Source: CAD feature listing. Evaluate the final solid. Frame: model axes, mm. A direction names the side the tool comes from. Give positions to 0.01 mm unless a question says otherwise; leave off trailing zeros. Order: outer loops, then holes, each group sorted by start corner. A loop starts at its lowest first (then second) coordinate and runs counter-clockwise, first axis right, second up. Notation, with made-up numbers: (35, 0.5) -> (75, 0.5) arc R30 ccw to (75, 30.5) -> close; hole circle Ø5 at (-37.75, -33). An arc over 180 degrees is marked (long way). Answer in a Markdown table with one row per item.
```python
from build123d import *

# Parameters (mm, degrees)
F0_W     = 57.15
F0_H     = 44.45
F1_DEPTH = 25.4
F2_W     = 44.45
F2_H     = 31.75
F3_DEPTH = 25.401
F5_DEPTH = 12.701
F7_DEPTH = 25.4


with BuildPart() as f1:
    # F0 (on Front) → F1 (new body)
    with BuildSketch(Plane.XZ):
        with Locations((-6.2023242936, 14.8889736688)):
            Rectangle(F0_W, F0_H)
    extrude(amount=F1_DEPTH)

    # F2 (on face) → F3 (cut, through all)
    with BuildSketch(Plane.XZ.offset(25.4)):
        with Locations((0.1476757064, 21.2389736688)):
            Rectangle(F2_W, F2_H)
    extrude(amount=-F3_DEPTH, mode=Mode.SUBTRACT)

    # F4 (on face) → F5 (cut, through all)
    with BuildSketch(Plane.XY.offset(5.3639736688)):
        with BuildLine():
            ThreePointArc((16.0226757064, -12.7), (14.1628037685, -8.209871941), (9.6726757108, -6.35))
            Line((9.6726757064, -6.35), (9.6726757064, -12.7))
            Line((9.6726757064, -12.7), (9.6726757064, -19.05))
            ThreePointArc((9.6726757179, -19.05), (14.162803771, -17.1901280565), (16.0226757064, -12.7))
        make_face()
        with BuildLine():
            ThreePointArc((9.6726757108, -6.35), (5.1825476475, -8.2098719379), (3.3226757064, -12.7))
            ThreePointArc((3.3226757064, -12.7), (5.18254765, -17.1901280646), (9.6726757179, -19.05))
            Line((9.6726757064, -19.05), (9.6726757064, -12.7))
            Line((9.6726757064, -12.7), (9.6726757064, -6.35))
        make_face()
        with BuildLine():
            ThreePointArc((-9.3773242936, -6.35), (-13.8674523541, -8.2098719395), (-15.7273242936, -12.7))
            ThreePointArc((-15.7273242936, -12.7), (-13.8674523541, -17.1901280605), (-9.3773242936, -19.05))
            ThreePointArc((-9.3773242936, -19.05), (-4.887196233, -17.1901280605), (-3.0273242936, -12.7))
            ThreePointArc((-3.0273242936, -12.7), (-4.887196233, -8.2098719395), (-9.3773242936, -6.35))
        make_face()
        with BuildLine():
            Line((16.0226757064, 0), (16.0226757064, -1.7014773719))
            ThreePointArc((16.0226757064, -1.7014773719), (18.6529318275, -3.7197438789), (20.6711983345, -6.35))
            Line((20.6711983345, -6.35), (22.3726757064, -6.35))
            Line((22.3726757064, -6.35), (22.3726757064, 0))
            Line((22.3726757064, 0), (16.0226757064, 0))
        make_face()
        with BuildLine():
            Line((16.0226757064, 0), (9.6726757064, 0))
            ThreePointArc((9.6726757064, 0), (12.9596775792, -0.4327420061), (16.0226757064, -1.7014773719))
            Line((16.0226757064, -1.7014773719), (16.0226757064, 0))
        make_face()
        with BuildLine():
            Line((22.3726757064, -6.35), (20.6711983345, -6.35))
            ThreePointArc((20.6711983345, -6.35), (21.9399337003, -9.4129981272), (22.3726757064, -12.7))
            Line((22.3726757064, -12.7), (22.3726757064, -6.35))
        make_face()
        with BuildLine():
            Line((22.3726757064, -19.05), (22.3726757064, -12.7))
            ThreePointArc((22.3726757064, -12.7), (21.9399337003, -15.9870018728), (20.6711983345, -19.05))
            Line((20.6711983345, -19.05), (22.3726757064, -19.05))
        make_face()
        with BuildLine():
            ThreePointArc((20.6711983345, -19.05), (18.6529318275, -21.6802561211), (16.0226757064, -23.6985226281))
            Line((16.0226757064, -23.6985226281), (16.0226757064, -25.4))
            Line((16.0226757064, -25.4), (22.3726757064, -25.4))
            Line((22.3726757064, -25.4), (22.3726757064, -19.05))
            Line((22.3726757064, -19.05), (20.6711983345, -19.05))
        make_face()
        with BuildLine():
            ThreePointArc((16.0226757064, -23.6985226281), (12.9596775792, -24.9672579939), (9.6726757064, -25.4))
            Line((9.6726757064, -25.4), (16.0226757064, -25.4))
            Line((16.0226757064, -25.4), (16.0226757064, -23.6985226281))
        make_face()
    extrude(amount=-F5_DEPTH, mode=Mode.SUBTRACT)

    # F6 (on face) → F7 (cut)
    with BuildSketch(Plane.YZ.offset(-22.0773242936)):
        with BuildLine():
            Line((-19.05, 30.7639736688), (-19.05, 24.4139736688))
            ThreePointArc((-19.05, 24.4139736688), (-17.1901280605, 28.9041017294), (-12.7, 30.7639736688))
            Line((-12.7, 30.7639736688), (-19.05, 30.7639736688))
        make_face()
        with BuildLine():
            Line((-6.35, 30.7639736688), (-12.7, 30.7639736688))
            ThreePointArc((-12.7, 30.7639736688), (-8.2098719395, 28.9041017294), (-6.35, 24.4139736688))
            Line((-6.35, 24.4139736688), (-6.35, 30.7639736688))
        make_face()
        with BuildLine():
            ThreePointArc((-12.7, 30.7639736688), (-17.1901280605, 28.9041017294), (-19.05, 24.4139736688))
            Line((-19.05, 24.4139736688), (-12.7, 24.4139736688))
            Line((-12.7, 24.4139736688), (-6.35, 24.4139736688))
            ThreePointArc((-6.35, 24.4139736688), (-8.2098719395, 28.9041017294), (-12.7, 30.7639736688))
        make_face()
        with BuildLine():
            Line((-19.05, 35.4124962969), (-19.05, 30.7639736688))
            Line((-19.05, 30.7639736688), (-12.7, 30.7639736688))
            Line((-12.7, 30.7639736688), (-6.35, 30.7639736688))
            Line((-6.35, 30.7639736688), (-6.35, 35.4124962969))
            ThreePointArc((-6.35, 35.4124962969), (-9.4129981272, 36.6812316627), (-12.7, 37.1139736688))
            ThreePointArc((-12.7, 37.1139736688), (-15.9870018728, 36.6812316627), (-19.05, 35.4124962969))
        make_face()
        with BuildLine():
            ThreePointArc((-23.6985226281, 30.7639736688), (-21.6802561211, 33.3942297899), (-19.05, 35.4124962969))
            Line((-19.05, 35.4124962969), (-19.05, 37.1139736688))
            Line((-19.05, 37.1139736688), (-25.4, 37.1139736688))
            Line((-25.4, 37.1139736688), (-25.4, 30.7639736688))
            Line((-25.4, 30.7639736688), (-23.6985226281, 30.7639736688))
        make_face()
        with BuildLine():
            ThreePointArc((-1.7014773719, 30.7639736688), (-0.4327420061, 27.7009755416), (0, 24.4139736688))
            Line((0, 24.4139736688), (0, 30.7639736688))
            Line((0, 30.7639736688), (-1.7014773719, 30.7639736688))
        make_face()
        with BuildLine():
            Line((-25.4, 30.7639736688), (-25.4, 24.4139736688))
            ThreePointArc((-25.4, 24.4139736688), (-24.9672579939, 27.7009755416), (-23.6985226281, 30.7639736688))
            Line((-23.6985226281, 30.7639736688), (-25.4, 30.7639736688))
        make_face()
        with BuildLine():
            Line((-19.05, 37.1139736688), (-19.05, 35.4124962969))
            ThreePointArc((-19.05, 35.4124962969), (-15.9870018728, 36.6812316627), (-12.7, 37.1139736688))
            Line((-12.7, 37.1139736688), (-19.05, 37.1139736688))
        make_face()
        with BuildLine():
            Line((-6.35, 37.1139736688), (-12.7, 37.1139736688))
            ThreePointArc((-12.7, 37.1139736688), (-9.4129981272, 36.6812316627), (-6.35, 35.4124962969))
            Line((-6.35, 35.4124962969), (-6.35, 37.1139736688))
        make_face()
        with BuildLine():
            Line((-6.35, 37.1139736688), (-6.35, 35.4124962969))
            ThreePointArc((-6.35, 35.4124962969), (-3.7197438789, 33.3942297899), (-1.7014773719, 30.7639736688))
            Line((-1.7014773719, 30.7639736688), (0, 30.7639736688))
            Line((0, 30.7639736688), (0, 37.1139736688))
            Line((0, 37.1139736688), (-6.35, 37.1139736688))
        make_face()
        with BuildLine():
            Line((-12.7, 24.4139736688), (-19.05, 24.4139736688))
            ThreePointArc((-19.05, 24.4139736688), (-17.1901280605, 19.9238456083), (-12.7, 18.0639736688))
            ThreePointArc((-12.7, 18.0639736688), (-8.2098719395, 19.9238456083), (-6.35, 24.4139736688))
            Line((-6.35, 24.4139736688), (-12.7, 24.4139736688))
        make_face()
    extrude(amount=-F7_DEPTH, mode=Mode.SUBTRACT)


solid = f1.part
```
(1) Section query D-D (x = -12.5). Return the cut outline in (y, z).
A:
| item | result |
|---|---|
| outline | (-25.4, -7.34) -> (-18.23, -7.34) -> (-18.23, 5.36) -> (-25.4, 5.36) -> close; (-7.17, -7.34) -> (0, -7.34) -> (0, 5.36) -> (-7.17, 5.36) -> close |
(2) Ray query, probe 1 along X at (y, z) = (-9.75, 2); probe 2 along Z at (x, y) = (-1.5, -0.75); probe 3 along X at (y, z) = (-1.25, 6). Return the intervals inside material, ascending.
A:
| item | result |
|---|---|
| probe 1 | x = -34.78 to -15, -3.75 to 4.05, 15.3 to 22.03 |
| probe 2 | z = -7.34 to 5.36 |
| probe 3 | x = -34.78 to -22.08 |
(3) First-contact query: pin 1 Ø10 at (y, z) = (-14, 27) entering from +X; pin 2 Ø12 at (x, y) = (11.5, -14.5) entering from +Z; pin 3 Ø9 at (x, z) = (-27.5, 32) entering from +Y; pin 4 Ø6 at (x, y) = (-26, -19.5) entering from +Z. Flat tips, straight axial feed; report the tip coordinate or a pass-through.
A:
| item | result |
|---|---|
| pin 1 | passes through |
| pin 2 | stops at z = 5.36 |
| pin 3 | stops at y = -0.38 |
| pin 4 | stops at z = 35.41 |
(4) Section query C-C (y = -8). Return the cut outline in (x, z), plus the area to 3 significant figures.
A:
| item | result |
|---|---|
| outline | (-34.78, -7.34) -> (-13.65, -7.34) -> (-13.65, 5.36) -> (-22.08, 5.36) -> (-22.08, 20.14) -> (-34.78, 20.14) -> close; (-5.11, -7.34) -> (5.4, -7.34) -> (5.4, 5.36) -> (-5.11, 5.36) -> close; (13.94, -7.34) -> (21.47, -7.34) -> (21.47, 5.36) -> (13.94, 5.36) -> close |
| area | 685 mm^2 |
(5) Section query A-A (z = -1). Return the cut outline in (x, y), plus the area to 3 significant figures.
A:
| item | result |
|---|---|
| outline | (-34.78, -25.4) -> (9.67, -25.4) arc R12.7 ccw to (9.67, 0) -> (-34.78, 0) -> close; hole circle Ø12.7 at (-9.38, -12.7); hole circle Ø12.7 at (9.67, -12.7) |
| area | 1,130 mm^2 |
(6) Access query for faces 5 (the flat face through (-34.777, -13, 9)), 6 (the flat face through (-22.077, -13, 17)). Directions: +Z, -Z, +X, -X, +Y, -Y. A direction counts if a zero-diameter tool reaches every point of the face in a straight line with its end or side. Return the directions, or none.
A:
| item | result |
|---|---|
| face 5 | +Z, -Z, -X, +Y, -Y |
| face 6 | +Z, +X, +Y, -Y |
(7) Pull-direction query (Y, two-part tool) for faces 1 (the flat face through (-28, -6.35, 30)), 2 (the flat face through (-28, -19.05, 30)), 3 (the flat face through (-18, 0, 5)), 4 (the flat face through (0, -13, 5.364)); classes: +Y half, -Y half, draft (parallel to the pull), parting line (faces both ways), or undercut.
A:
| item | result |
|---|---|
| face 1 | undercut |
| face 2 | undercut |
| face 3 | +Y half |
| face 4 | draft |
(8) Section query B-B (x = -29). Return the cut outline in (y, z).
A:
| item | result |
|---|---|
| outline | (-25.4, -7.34) -> (0, -7.34) -> (0, 24.41) arc R12.7 ccw to (-6.35, 35.41) -> (-6.35, 24.41) arc R6.35 cw to (-19.05, 24.41) -> (-19.05, 35.41) arc R12.7 ccw to (-25.4, 24.41) -> close |
